For this review, take the finished solid that the model builds, in its own axes (mm). A direction names the side the tool comes from. Round coordinates to 2 decimals unless told otherwise and drop trailing zeros. Write each loop counter-clockwise with the first axis right and the second up, starting at its lowest first coordinate (ties: lowest second). Pieces come first, ordered by that corner, then holes. Notation, with made-up numbers: M -10.5,54 L -6.5,54 A30 cw -6.5,90 Z; hole C 81.25,23 d8. An arc over 180 degrees is marked long. Answer in a Markdown table with one row per item.
Autodesk Inventor part; units mm, degrees
ref_plane "YZ Plane" through (0, 0, 0) normal (1, 0, 0) x (0, 1, 0)
ref_plane "XZ Plane" through (0, 0, 0) normal (0, 1, 0) x (-1, 0, 0)
ref_plane "XY Plane" through (0, 0, 0) normal (0, 0, 1) x (1, 0, 0)
sketch "Skizze1" plane through (0, 0, 0) normal (0, 0, 1) x (1, 0, 0)
  line L0 (1.4434, 2.5) -> (2.8868, 0)
  line L1 (2.8868, 0) -> (1.4434, -2.5)
  line L2 (1.4434, -2.5) -> (-1.4434, -2.5)
  line L3 (-1.4434, -2.5) -> (-2.8868, 0)
  line L4 (-2.8868, 0) -> (-1.4434, 2.5)
  line L5 (-1.4434, 2.5) -> (1.4434, 2.5)
  point P0 (0, 0)
  point P1 (0, 0)
  dimension "d0" = 5
extrude "Extrusion1" add sketch "Skizze1" along normal blind 5
sketch "Skizze2" plane through (0, 0, 0) normal (0, 0, -1) x (-1, 0, 0)
  circle A0 centre (0, 0) radius 1.25
  dimension "d3" = 2.5
extrude "Extrusion2" add sketch "Skizze2" along normal blind 4
chamfer "Fasen1" distance 0.2 angle 45 1 edges at (1.25, 0, -4)
sketch "Skizze3" plane through (0, 0, 5) normal (0, 0, 1) x (1, 0, 0)
  point P0 (0, 0)
  point P1 (0, 0)
hole "Bohrung1" at (0, 0, 5) direction (0, 0, -1) diameter 2.013 depth 3 tip angle 118
thread "Gewinde1"
chamfer "Fasen2" distance 0.2 angle 45 12 edges at (2.1651, 1.25, 5) (2.1651, -1.25, 5) (0, -2.5, 5) (-2.1651, -1.25, 5) (-2.1651, 1.25, 5) (0, 2.5, 5) (0, 2.5, 0) (2.1651, 1.25, 0) (2.1651, -1.25, 0) (-2.1651, 1.25, 0) (-2.1651, -1.25, 0) (0, -2.5, 0)
properties part number "Abstandsbolzen_Jetson"
Q1. Machinability: for faces 4 (the face through (0.983, 0.218, 3.479)), 5 (the face through (1, 1, 5)), 6 (the face through (0.27, 1.22, -1.87)), which of the approach directions +Z, -Z, +X, -X, +Y, -Y give a long, thin tool a straight path to every point of the face, cutting with its end or side? Answer none if there is none.
Found:
| item | result |
|---|---|
| face 4 | +Z |
| face 5 | +Z, +X, -X, +Y, -Y |
| face 6 | -Z |
Q2. Take a section at B-B (x = -2.35). State the section outline as (y, z) points, then the cut area to 3 significant figures.
Found:
| item | result |
|---|---|
| outline | M -0.93,0.2 L -0.53,0 L 0.53,0 L 0.93,0.2 L 0.93,4.8 L 0.53,5 L -0.53,5 L -0.93,4.8 Z |
| area | 9.14 mm² |
Q3. Take a section at A-A (z = 2.25). State the section outline as (x, y) points, then the cut area to 3 significant figures.
Found:
| item | result |
|---|---|
| outline | M -2.89,0 L -1.44,-2.5 L 1.44,-2.5 L 2.89,0 L 1.44,2.5 L -1.44,2.5 Z; hole C 0,0 d2.01 |
| area | 18.5 mm² |
Q4. Mouldability with a two-part tool opening along Y and no side actions: class faces 1 (the face through (0.05, -0.17, 1.5)), 2 (the face through (1, 1, 0)), 3 (the face through (2.175, -1.233, 2.468)) as +Y half, -Y half, draft (parallel to the pull), parting line (faces both ways), or undercut.
Found:
| item | result |
|---|---|
| face 1 | undercut |
| face 2 | draft |
| face 3 | -Y half |
Q5. Insertion check: P1, Ø1.2, axis at x = 0, y = 0, coming from the +Z side; P2, Ø3, axis at x = -0.5, y = 1, coming from the -Z side; P3, Ø1.5, axis at x = -2.5, z = -3, coming from the +Y side; P4, Ø1.5, axis at x = 1, z = -1, coming from the +Y side. Each pin has a flat end and moves straight along its axis. Give the tip position at first contact, or say it passes through.
Found:
| item | result |
|---|---|
| P1 | z = 1.76 |
| P2 | z = -4 |
| P3 | through |
| P4 | y = 1.22 |
Q6. For probe 1 along Y at (x, z) = (0, 3.7); probe 2 along Z at (x, y) = (0.2, -1.45); probe 3 along Z at (x, y) = (0, 0.3), list the stretches that pass through material, from the lowest coordinate up.
Found:
| item | result |
|---|---|
| probe 1 | -2.5 to -1.01, 1.01 to 2.5 |
| probe 2 | 0 to 5 |
| probe 3 | -4 to 1.58 |
Q7. Take a section at C-C (x = -1.6). State the section outline as (y, z) points, then the cut area to 3 significant figures.
Found:
| item | result |
|---|---|
| outline | M -2.23,0.2 L -1.83,0 L 1.83,0 L 2.23,0.2 L 2.23,4.8 L 1.83,5 L -1.83,5 L -2.23,4.8 Z |
| area | 22.1 mm² |
